```python
from build123d import *

# Parameters (mm, degrees)
F1_DEPTH = 44
F2_R     = 2.5
F2_R_2   = 2.779494
F2_R_3   = 3.003014
F3_DEPTH = 2.748387
F5_DEPTH = 4
F7_DEPTH = 4


with BuildPart() as f1:
    # F0 (on Front) → F1 (new body, symmetric)
    with BuildSketch(Plane.XZ):
        Polygon((33.024074, -6.624926), (-2.974825, -6.624926), (-2.974825, -9.624926), (36.025175, -9.624926), (36.025175, 62.375074), (48.024074, 62.375074), (48.024074, 65.123461), (33.024074, 65.123461), align=None)
        Polygon((-2.974825, -9.624926), (-2.974825, -6.624926), (-38.973723, -6.624926), (-38.973723, 65.123461), (-53.973723, 65.123461), (-53.973723, 62.375074), (-41.974825, 62.375074), (-41.974825, -9.624926), align=None)
    extrude(amount=F1_DEPTH, both=True)

    # F2 (on face) → F3 (cut, through all)
    with BuildSketch(Plane.XY.offset(65.123461)):
        with Locations((42.024624, -29)):
            Circle(F2_R)
        with Locations((42.024624, 29)):
            Circle(F2_R)
        with Locations((-47.974274, 29)):
            Circle(F2_R)
        with Locations((-47.974274, -29)):
            Circle(F2_R)
        with Locations((-47.974274, 0.645779)):
            Circle(F2_R_2)
        with Locations((42.024624, 0)):
            Circle(F2_R_3)
    extrude(amount=-F3_DEPTH, mode=Mode.SUBTRACT)

    # F4 (on face) → F5 (cut)
    with BuildSketch(Plane(origin=(0, 0, -9.624926), x_dir=(1, 0, 0), z_dir=(0, 0, -1))):
        Polygon((-1.577392, 3.848274), (24.135478, 29.56114), (-29.805643, 28.443189), align=None)
        Polygon((24.135478, -29.131273), (-1.577392, -7.890209), (-29.805643, -29.131273), align=None)
    extrude(amount=-F5_DEPTH, mode=Mode.SUBTRACT)

    # F6 (on face) → F7 (cut)
    with BuildSketch(Plane.YZ.offset(36.025175)):
        Polygon((29.453758, 16.755113), (29.453758, 58.549069), (-31.596411, 37.797935), align=None)
    extrude(amount=-F7_DEPTH, mode=Mode.SUBTRACT)


solid = f1.part
```
Here's how the part is built. I have some questions about the finished solid (model axes, mm). A direction names the side the tool comes from. Coordinates: 2 decimals unless noted, no trailing zeros. Write each loop counter-clockwise with the first axis right and the second up, starting at its lowest first coordinate (ties: lowest second). Pieces come first, ordered by that corner, then holes. Notation, with made-up numbers: (80, 30) -> (138, 30) arc R27 ccw to (138, 50) -> close; hole circle Ø8 at (-25, 28.25). An arc over 180 degrees is marked (long way). Use a Markdown table: item, result. Add a question column.
(1) For faces 4 (the flat face through (33.024, -1, 22)), 5 (the flat face through (35, 29.454, 37)), 6 (the flat face through (-41.975, -1, 27)), 7 (the flat face through (11.099, -16.525, -8.146)), which set-ups out of +Z, -Z, +X, -X, +Y, -Y let a thin tool reach every point of the face, with its end or its side?
(2) If we section it at B-B, the plane x = -3: Write out the boundary of the cut face in (y, z), and give its area (3 significant figures).
(3) If we section it at D-D, the plane z = 23.5: Write out the boundary of the cut face in (x, y), and give its area (3 significant figures).
(4) Please list where these lines run through material, in increasing order: line 1 (X direction, y = 12.5, z = -0.5); line 2 (Z direction, x = 18.5, y = -8.5); line 3 (Z direction, x = 42.5, y = 35.5).
(5) We'd pull the mould along Y, two halves only. Please class faces 1 (the flat face through (34.55, -0.64, 48.32)), 2 (the flat face through (-3, 44, -8)), 3 (the flat face through (-45, -1, 62.375)): +Y half, -Y half, draft (parallel to the pull), parting line (faces both ways), or undercut.
(6) I'm going to push flat-ended pins straight in: P1, Ø1, axis at y = -18.5, z = 2.5, coming from the -X side; P2, Ø4, axis at y = 5.5, z = 8.5, coming from the +X side; P3, Ø6.5, axis at x = -47.97, y = -29, coming from the -Z side; P4, Ø4, axis at x = 42.02, y = -29, coming from the +Z side. Where does each tip first touch, or does it pass through?
(7) If we section it at A-A, the plane z = 13: Write out the boundary of the cut face in (x, y).
(8) If we section it at C-C, the plane y = 33: Write out the boundary of the cut face in (x, z), and give its area (3 significant figures).
Outcome:
| question | item | result |
|---|---|---|
| 1 | face 4 | +Z, +Y, -Y |
| 1 | face 5 | +X |
| 1 | face 6 | -Z, -X, +Y, -Y |
| 1 | face 7 | +Z, -Z |
| 2 | outline | (-44, -9.62) -> (-29, -9.62) -> (-29, -6.62) -> (-44, -6.62) -> close; (-5.09, -9.62) -> (8.96, -9.62) -> (8.96, -6.62) -> (-5.09, -6.62) -> close; (29.13, -9.62) -> (44, -9.62) -> (44, -6.62) -> (29.13, -6.62) -> close |
| 2 | area | 132 mm^2 |
| 3 | outline | (-41.97, -44) -> (-38.97, -44) -> (-38.97, 44) -> (-41.97, 44) -> close; (33.02, -44) -> (36.03, -44) -> (36.03, 9.89) -> (33.02, 9.89) -> close; (33.02, 29.45) -> (36.03, 29.45) -> (36.03, 44) -> (33.02, 44) -> close |
| 3 | area | 469 mm^2 |
| 4 | line 1 | x = -41.97 to -38.97, 33.02 to 36.03 |
| 4 | line 2 | z = -9.62 to -6.62 |
| 4 | line 3 | z = 62.38 to 65.12 |
| 5 | face 1 | undercut |
| 5 | face 2 | +Y half |
| 5 | face 3 | draft |
| 6 | P1 | stops at x = -41.97 |
| 6 | P2 | stops at x = 36.03 |
| 6 | P3 | stops at z = 62.38 |
| 6 | P4 | passes through |
| 7 | outline | (-41.97, -44) -> (-38.97, -44) -> (-38.97, 44) -> (-41.97, 44) -> close; (33.02, -44) -> (36.03, -44) -> (36.03, 44) -> (33.02, 44) -> close |
| 8 | outline | (-53.97, 62.38) -> (-41.97, 62.38) -> (-41.97, -9.62) -> (36.03, -9.62) -> (36.03, 62.38) -> (48.02, 62.38) -> (48.02, 65.12) -> (33.02, 65.12) -> (33.02, -6.62) -> (-38.97, -6.62) -> (-38.97, 65.12) -> (-53.97, 65.12) -> close |
| 8 | area | 731 mm^2 |
